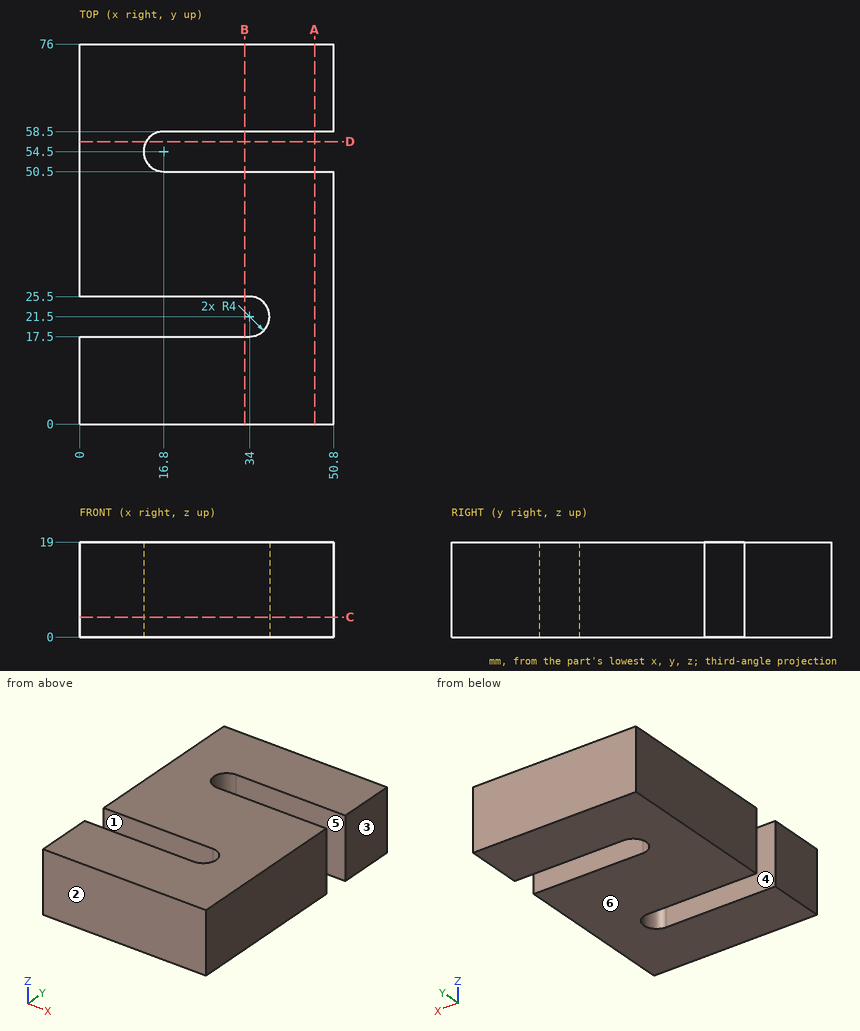
Design review of the part shown in the three views and the two pictorial views. Dimensions are in mm from the part's minimum x, y and z. A direction names the side the tool comes from. Give positions to 0.01 mm unless a question says otherwise; leave off trailing zeros. Write each loop counter-clockwise with the first axis right and the second up, starting at its lowest first coordinate (ties: lowest second). Pieces come first, ordered by that corner, then holes.
Item 1: Wall thickness on probe 1 along Y at (x, z) = (16.5, 3); probe 2 along Y at (x, z) = (43, 8.5); probe 3 along Y at (x, z) = (16, 12.75): over which ranges is each line inside the solid? List them lowest first.
Item 2: Take a section at B-B (x = 33). Give the boundary of the cut face in (y, z).
Item 3: The part is to be moulded in two halves that separate along Y. For the marked faces 1, 2 and 3, say which applies: +Y half, -Y half, draft (parallel to the pull), parting line (faces both ways), or undercut.
Item 4: Take a section at D-D (y = 56.5). Give the boundary of the cut face in (x, z).
Item 5: Take a section at C-C (z = 4). Give the boundary of the cut face in (x, y).
Item 6: Machinability: for the marked faces 4, 5 and 6, which of the approach directions +Z, -Z, +X, -X, +Y, -Y give a long, thin tool a straight path to every point of the face, cutting with its end or side? Answer none if there is none.
Item 7: Take a section at A-A (x = 47). Give the boundary of the cut face in (y, z).
Established:
1. probe 1: y = 0 to 17.5, 25.5 to 50.51, 58.49 to 76
1. probe 2: y = 0 to 50.5, 58.5 to 76
1. probe 3: y = 0 to 17.5, 25.5 to 50.58, 58.42 to 76
2. outline: (0, 0) - (17.5, 0) - (17.5, 19) - (0, 19) - close; (25.5, 0) - (50.5, 0) - (50.5, 19) - (25.5, 19) - close; (58.5, 0) - (76, 0) - (76, 19) - (58.5, 19) - close
3. face 1: undercut
3. face 2: -Y half
3. face 3: draft
4. outline: (0, 0) - (13.34, 0) - (13.34, 19) - (0, 19) - close
5. outline: (0, 0) - (50.8, 0) - (50.8, 50.5) - (16.8, 50.5) arc R4 cw to (16.8, 58.5) - (50.8, 58.5) - (50.8, 76) - (0, 76) - (0, 25.5) - (34, 25.5) arc R4 cw to (34, 17.5) - (0, 17.5) - close
6. face 4: +Z, -Z, -X
6. face 5: +Z, -Z, +X
6. face 6: -Z, +X, -X, +Y, -Y
7. outline: (0, 0) - (50.5, 0) - (50.5, 19) - (0, 19) - close; (58.5, 0) - (76, 0) - (76, 19) - (58.5, 19) - close
